```python
from build123d import *

# Parameters (mm, degrees)
BOSS_EXTRUDE1_DEPTH                 = 177.8
F_9_64_0_14063_DIAMETER_HOLE1_D     = 3.572002
F_9_64_0_14063_DIAMETER_HOLE1_DEPTH = 2.54
CUT_EXTRUDE1_START                  = -2.54
CUT_EXTRUDE1_DEPTH                  = 2.54
LPATTERN1_COUNT                     = 9
LPATTERN1_PITCH                     = 19.05


# Read off the part's stored shape, not the designer's step: Cut-Extrude1
with BuildPart() as part:
    # Sketch2 → Boss-Extrude1 (new body)
    with BuildSketch(Plane(origin=(0, 0, 0), x_dir=(0, 0, -1), z_dir=(1, 0, 0))):
        Polygon((-6.35, 0), (6.35, 0), (6.35, 7.62), (1.27, 7.62), (1.27, 6.35), (5.08, 6.35), (5.08, 2.54), (-5.08, 2.54), (-5.08, 6.35), (-1.27, 6.35), (-1.27, 7.62), (-6.35, 7.62), align=None)
    extrude(amount=BOSS_EXTRUDE1_DEPTH)

    # 9/64 (0.14063) Diameter Hole1
    with Locations(Plane(origin=(0, 2.54, 0), x_dir=(-1, 0, 0), z_dir=(0, 1, 0))):
        with Locations((-3.302, 0), (-174.498, 0)):
            Hole(F_9_64_0_14063_DIAMETER_HOLE1_D / 2, depth=F_9_64_0_14063_DIAMETER_HOLE1_DEPTH)

    # Cut-Extrude1 outline → Cut-Extrude1 (cut)
    with BuildSketch(Plane(origin=(0, 2.54, 0), x_dir=(1, 0, 0), z_dir=(0, 1, 0)).offset(CUT_EXTRUDE1_START)):
        with BuildLine():
            Line((15.875, 3.175), (9.525, 3.175))
            ThreePointArc((9.525, 3.175), (6.35, 0), (9.525, -3.175))
            Line((9.525, -3.175), (15.875, -3.175))
            ThreePointArc((15.875, -3.175), (19.05, 0), (15.875, 3.175))
        make_face()
    cut_extrude1 = extrude(amount=CUT_EXTRUDE1_DEPTH, mode=Mode.SUBTRACT)

    # LPattern1: Cut-Extrude1 ×9
    with Locations(*[(i * LPATTERN1_PITCH, 0, 0) for i in range(1, LPATTERN1_COUNT)]):
        add(cut_extrude1, mode=Mode.SUBTRACT)


solid = part.part
```
Read the model definition and answer for the solid it produces. Units are mm, in the model's axes. A direction names the side the tool comes from. Give positions to 0.01 mm unless a question says otherwise; leave off trailing zeros. Loops run counter-clockwise (first coordinate to the right, second up) from the corner with the lowest first, then second, coordinate; pieces in that order, holes last.
Item 1: The part is cut by section B-B (x = 12). Write down the section's boundary in (y, z) (3 decimals), and give its area (3 significant figures).
Item 2: The mould has two halves that part along Y. Classify faces 4 (the flat face through (88, 0, -4)), 5 (the cylindrical face through (82.55, 1.25, -0.07)), 6 (the flat face through (87.7, 2.54, -3.5)): released by +Y, released by -Y, zero draft, split by the parting line, or undercut.
Item 3: Find the intervals of material crossed by line 1 along Z through (x, y) = (86, 2.75); line 2 along Y through (x, z) = (129.5, -3.5); line 3 along Z through (x, y) = (72, 1.75) (3 decimals), in increasing order.
Item 4: For faces 1 (the flat face through (88, 6.35, 3)), 2 (the cylindrical face through (19.05, 1.25, 0.07)), 3 (the flat face through (88, 7.62, 4)), determine the directions among +Z, -Z, +X, -X, +Y, -Y from which every point of the face is accessible in a straight line to the end or side of a thin tool.
Item 5: The part is cut by section C-C (x = 137.5). Write down the section's boundary in (y, z).
Item 6: The part is cut by section A-A (y = 3.75). Write down the section's boundary in (x, z).
Taken from the geometry:
1. outline: (0, -6.35) - (7.62, -6.35) - (7.62, -1.27) - (6.35, -1.27) - (6.35, -5.08) - (2.54, -5.08) - (2.54, -3.175) - (0, -3.175) - close; (0, 3.175) - (2.54, 3.175) - (2.54, 5.08) - (6.35, 5.08) - (6.35, 1.27) - (7.62, 1.27) - (7.62, 6.35) - (0, 6.35) - close
1. area: 38.7 mm2
2. face 4: released by -Y
2. face 5: zero draft
2. face 6: undercut
3. line 1: z = -6.35 to -5.08, 5.08 to 6.35
3. line 2: y = 0 to 2.54, 6.35 to 7.62
3. line 3: z = -6.35 to -3.175, 3.175 to 6.35
4. face 1: +X, -X
4. face 2: -Y
4. face 3: +Z, -Z, +X, -X, +Y
5. outline: (0, -6.35) - (7.62, -6.35) - (7.62, -1.27) - (6.35, -1.27) - (6.35, -5.08) - (2.54, -5.08) - (2.54, 5.08) - (6.35, 5.08) - (6.35, 1.27) - (7.62, 1.27) - (7.62, 6.35) - (0, 6.35) - close
6. outline: (0, -6.35) - (177.8, -6.35) - (177.8, -5.08) - (0, -5.08) - close; (0, 5.08) - (177.8, 5.08) - (177.8, 6.35) - (0, 6.35) - close
